Source: three-view drawing plus pictorial views. Frame: mm from the lowest corner of the part. Give positions to 0.01 mm unless a question says otherwise; leave off trailing zeros. Order: outer loops, then holes, each group sorted by start corner. A loop starts at its lowest first (then second) coordinate and runs counter-clockwise, first axis right, second up. Notation, with made-up numbers: M 26.25,84.5 L 44.25,84.5 A16 cw 44.25,109.5 Z; hole C -22.5,-37.5 d6. An arc over 180 degrees is marked long. Use CSV: the item, a comma, the result in double quotes. Start each with the question number.
1. Section query C-C, the plane z = 60. Return the cut outline in (x, y) (3 decimals), plus the area to 3 significant figures.
2. Mould query, pull axis Y, two halves, no side actions, for the marked faces 1, 2, 3 and 4. Classes: released by +Y, released by -Y, zero draft, split by the parting line, or undercut.
3. Pin query (flat end, axial travel): P1, Ø1.5, axis at x = 18, z = 44, coming from the -Y side (3 decimals). Return the tip coordinate at first contact, or that it passes through.
4. Section query B-B, the plane y = 13. Return the cut outline in (x, z) (3 decimals), plus the area to 3 significant figures.
5. Section query D-D, the plane z = 24. Return the cut outline in (x, y) (3 decimals), plus the area to 3 significant figures.
6. Line query: line 1 along Y through (x, z) = (9, 62.5) (3 decimals); line 2 along X through (y, z) = (9, 45) (3 decimals); line 3 along Y through (x, z) = (15, 47) (3 decimals). Output: solid intervals per line, ascending. Write a range as [from, to].
7. Section query A-A, the plane x = 14.75. Return the cut outline in (y, z) (3 decimals).
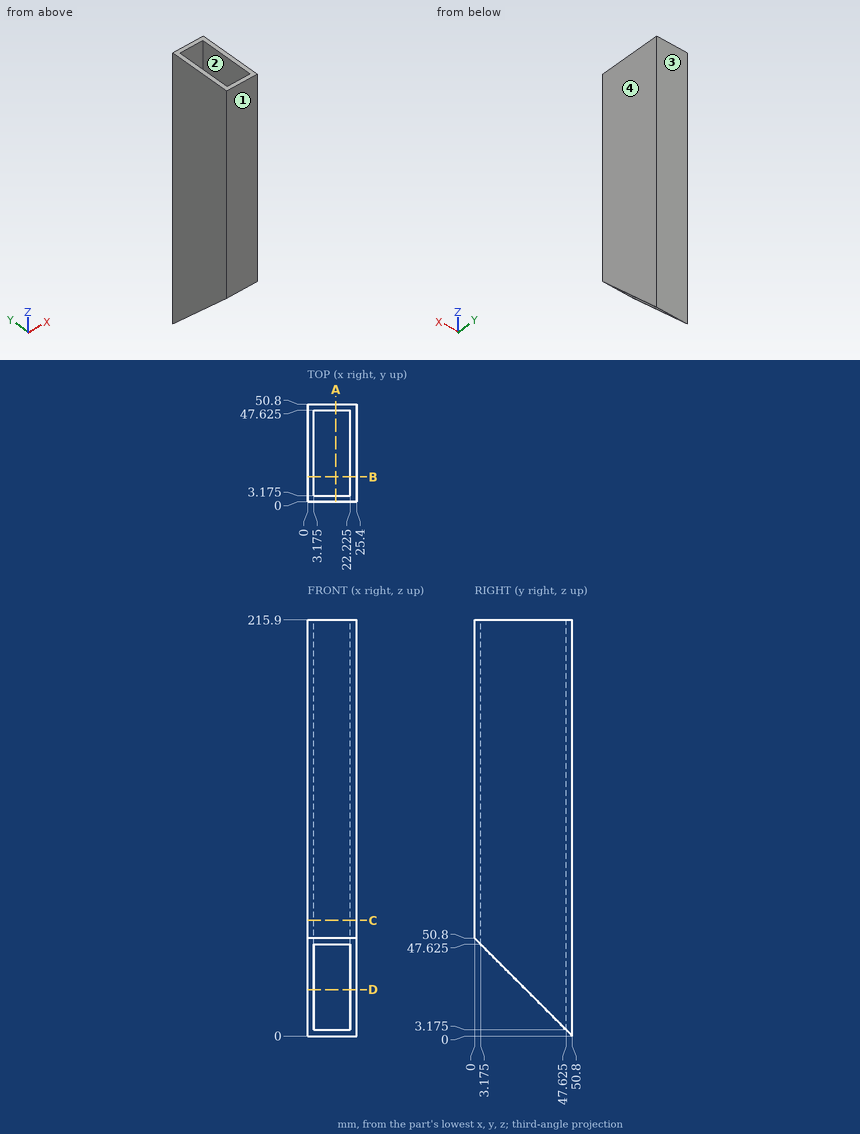
Result set:
1,outline,"M 0,0 L 25.4,0 L 25.4,50.8 L 0,50.8 Z; hole M 3.175,3.175 L 22.225,3.175 L 22.225,47.625 L 3.175,47.625 Z"
1,area,"444 mm2"
2,face 1,"released by -Y"
2,face 2,"undercut"
2,face 3,"released by +Y"
2,face 4,"zero draft"
3,P1,"y = 47.625"
4,outline,"M 0,37.8 L 3.175,37.8 L 3.175,215.9 L 0,215.9 Z; M 22.225,37.8 L 25.4,37.8 L 25.4,215.9 L 22.225,215.9 Z"
4,area,"1,130 mm2"
5,outline,"M 0,26.8 L 3.175,26.8 L 3.175,47.625 L 22.225,47.625 L 22.225,26.8 L 25.4,26.8 L 25.4,50.8 L 0,50.8 Z"
5,area,"213 mm2"
6,line 1,"[0, 3.175], [47.625, 50.8]"
6,line 2,"[0, 3.175], [22.225, 25.4]"
6,line 3,"[47.625, 50.8]"
7,outline,"M 0,50.8 L 3.175,47.625 L 3.175,215.9 L 0,215.9 Z; M 47.625,3.175 L 50.8,0 L 50.8,215.9 L 47.625,215.9 Z"
